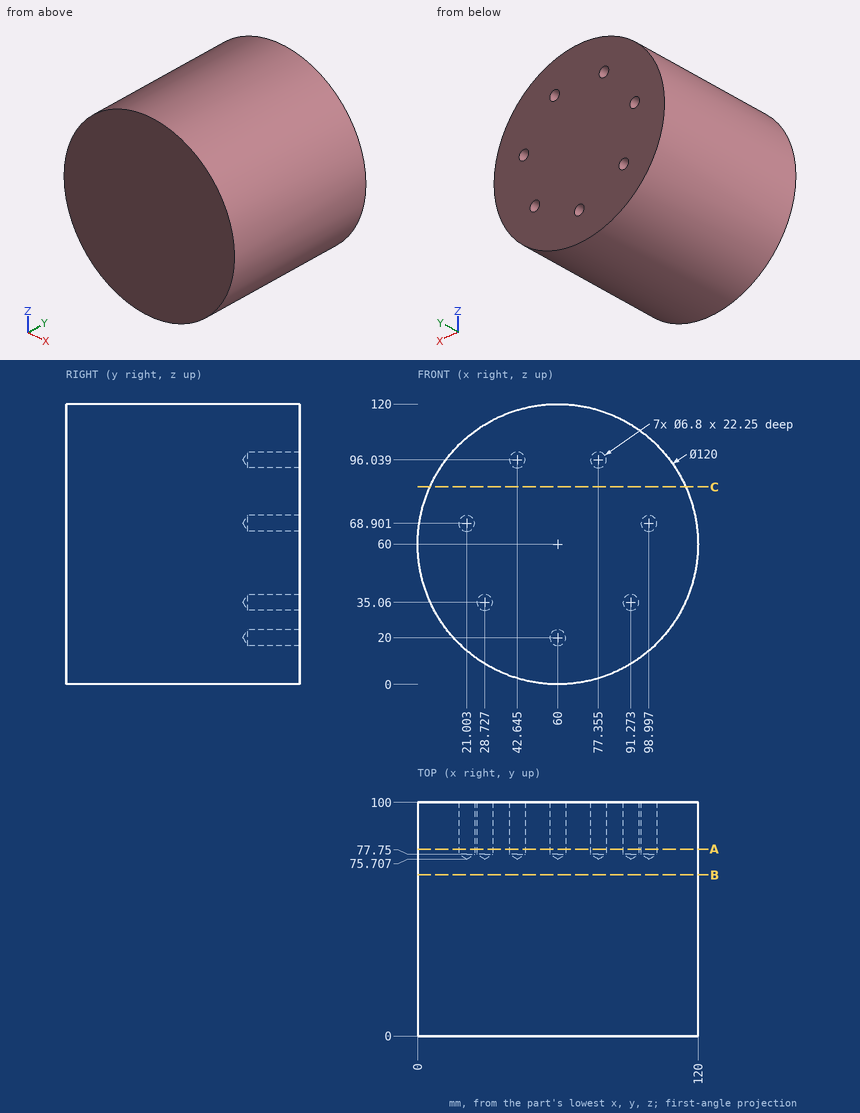
Study the drawing (mm; zero at the part's minimum x, y, z) and answer. Coordinates: 2 decimals unless noted, no trailing zeros. Write each loop counter-clockwise with the first axis right and the second up, starting at its lowest first coordinate (ties: lowest second). Pieces come first, ordered by that corner, then holes.
Q1. Each of these flat-tipped pins is pushed along its axis until it touches: pin 1 Ø5.5 at (x, z) = (99, 68.9) entering from +Y; pin 2 Ø8 at (x, z) = (42.64, 96.04) entering from +Y; pin 3 Ø12 at (x, y) = (22.5, 88) entering from +Z (1 decimal); pin 4 Ø12 at (y, z) = (19.5, 69.5) entering from -X. Where does it stop, or does it pass through?
Q2. A cutting plane is placed at A-A, the plane y = 80. Give the vertices of the cut face in (x, z) (1 decimal).
Q3. A cutting plane is placed at C-C, the plane z = 84.5. Give the vertices of the cut face in (x, y), then the cut area to 3 significant figures.
Q4. A cutting plane is placed at B-B, the plane y = 69. Give the vertices of the cut face in (x, z).
Q5. Find the intervals of material crossed by line 1 (Z direction, x = 62, y = 16); line 2 (X direction, y = 73.5, z = 64); line 3 (X direction, y = 20.5, z = 67.5), in increasing order.
Findings below:
1. pin 1: stops at y = 77.36
1. pin 2: stops at y = 100
1. pin 3: stops at z = 111.1
1. pin 4: stops at x = 0.1
2. outline: circle Ø120 at (60, 60); hole circle Ø6.8 at (21, 68.9); hole circle Ø6.8 at (28.7, 35.1); hole circle Ø6.8 at (42.6, 96); hole circle Ø6.8 at (60, 20); hole circle Ø6.8 at (77.4, 96); hole circle Ø6.8 at (91.3, 35.1); hole circle Ø6.8 at (99, 68.9)
3. outline: (5.23, 0) - (114.77, 0) - (114.77, 100) - (5.23, 100) - close
3. area: 11,000 mm2
4. outline: circle Ø120 at (60, 60)
5. line 1: z = 0.03 to 119.97
5. line 2: x = 0.13 to 119.87
5. line 3: x = 0.47 to 119.53
